Can you work these out from the model? Positions are in its coordinate system, mm. A direction names the side the tool comes from. Coordinates: 2 decimals unless noted, no trailing zeros. Order: outer loops, then holes, each group sorted by start corner. A loop starts at its lowest first (then second) coordinate and runs counter-clockwise, first axis right, second up. Notation, with made-up numbers: (-38, 41.25) -> (-16, 41.25) arc R36 cw to (-16, 75.25) -> close; hole circle Ø1 at (59, 36.5). An arc over 180 degrees is marked (long way). Return JSON: item names as keys, results as strings. Group by question number.
1) For pin 1 (8 mm diameter, centred on x = -94.5, y = 19, fed in from -Z); pin 2 (8 mm diameter, centred on y = 14.5, z = -120.5, fed in from -X); pin 3 (1.5 mm diameter, centred on x = -74.5, z = -125.5, fed in from -Y), each with a flat end and sliding along its axis, tell me the tip position at first contact or that it passes through.
2) Thinking about a two-plate mould opening in X: for faces 4 (the cylindrical face through (-73.365, 15.077, -118.443)), 5 (the flat face through (-70.9, 11, -122)), 6 (the cylindrical face through (-87.404, 15.154, -104.477)), 7 (the flat face through (-110.9, 15, -103)), which applies, +X half, -X half, draft (parallel to the pull), parting line (faces both ways), or undercut?
3) If we section it at B-B, the plane z = -124.5: Please give me the cut outline in (x, y).
4) For faces 1 (the flat face through (-75.9, 11, -125)), 2 (the flat face through (-72, 15, -141.942)), 3 (the flat face through (-73, 11.5, -127)), which set-ups out of +Z, -Z, +X, -X, +Y, -Y let a thin tool reach every point of the face, with its end or its side?
5) If we section it at A-A, the plane y = 15: Please give me the cut outline in (x, z).
6) If we section it at C-C, the plane x = -90.5: Please give me the cut outline in (y, z).
7) If we section it at D-D, the plane y = 8.5: Please give me the cut outline in (x, z), then the cut area to 3 significant figures.
8) If I drill on probe 1 along Z at (x, y) = (-73, 5.25); probe 2 along Z at (x, y) = (-88.5, 22); probe 3 along X at (y, z) = (7.75, -111.5), over which ranges is the centre line in solid material (lowest first)? Write a range as from..to.
from build123d import *

# Parameters (mm, degrees)
F1_DEPTH = 30
F3_D     = 7
F5_DEPTH = 25


with BuildPart() as f1:
    # F0 (on Front) → F1 (new body)
    with BuildSketch(Plane.XZ):
        with BuildLine():
            ThreePointArc((-80.400344, -106.942194), (-77.515036, -107.988935), (-75.972026, -110.642194))
            ThreePointArc((-75.972026, -110.642194), (-75.9183, -111.040591), (-75.900344, -111.442194))
            Line((-75.900344, -111.442194), (-75.900344, -138.942194))
            ThreePointArc((-75.900344, -138.942194), (-75.021664, -141.063514), (-72.900344, -141.942194))
            Line((-72.900344, -141.942194), (-70.900344, -141.942194))
            Line((-70.900344, -141.942194), (-70.900344, -101.942194))
            Line((-70.900344, -101.942194), (-110.900344, -101.942194))
            Line((-110.900344, -101.942194), (-110.900344, -103.942194))
            ThreePointArc((-110.900344, -103.942194), (-110.021664, -106.063514), (-107.900344, -106.942194))
            Line((-107.900344, -106.942194), (-80.400344, -106.942194))
        make_face()
    extrude(amount=-F1_DEPTH)

    # F3 (through all)
    with Locations(Plane.XY.offset(-101.942194)):
        with Locations((-90.900344, 15)):
            Hole(F3_D / 2)

    # F4 (on face) → F5 (cut)
    with BuildSketch(Plane.YZ.offset(-70.900344)):
        with BuildLine():
            ThreePointArc((11.5, -131.942194), (15, -135.442194), (18.5, -131.942194))
            Line((18.5, -131.942194), (18.5, -121.942194))
            ThreePointArc((18.5, -121.942194), (15, -118.442194), (11.5, -121.942194))
            Line((11.5, -121.942194), (11.5, -131.942194))
        make_face()
    extrude(amount=-F5_DEPTH, mode=Mode.SUBTRACT)


solid = f1.part
Result sheet:
{
 "1": {"pin 1": "stops at z = -106.94", "pin 2": "stops at x = -75.9", "pin 3": "stops at y = 0"},
 "2": {"face 4": "draft", "face 5": "+X half", "face 6": "undercut", "face 7": "-X half"},
 "3": {"outline": "(-75.9, 0) -> (-70.9, 0) -> (-70.9, 11.5) -> (-75.9, 11.5) -> close; (-75.9, 18.5) -> (-70.9, 18.5) -> (-70.9, 30) -> (-75.9, 30) -> close"},
 "4": {"face 1": "-Z, -X, +Y, -Y", "face 2": "-Z, +X, -X, +Y, -Y", "face 3": "+X, -X"},
 "5": {"outline": "(-110.9, -103.94) arc R3 ccw to (-107.9, -106.94) -> (-94.4, -106.94) -> (-94.4, -101.94) -> (-110.9, -101.94) -> close; (-87.4, -106.94) -> (-80.4, -106.94) arc R4.5 cw to (-75.97, -110.64) arc R4.5 cw to (-75.9, -111.44) -> (-75.9, -118.44) -> (-70.9, -118.44) -> (-70.9, -101.94) -> (-87.4, -101.94) -> close; (-75.9, -138.94) arc R3 ccw to (-72.9, -141.94) -> (-70.9, -141.94) -> (-70.9, -135.44) -> (-75.9, -135.44) -> close"},
 "6": {"outline": "(0, -106.94) -> (11.52, -106.94) -> (11.52, -101.94) -> (0, -101.94) -> close; (18.48, -106.94) -> (30, -106.94) -> (30, -101.94) -> (18.48, -101.94) -> close"},
 "7": {"outline": "(-110.9, -103.94) arc R3 ccw to (-107.9, -106.94) -> (-80.4, -106.94) arc R4.5 cw to (-75.97, -110.64) arc R4.5 cw to (-75.9, -111.44) -> (-75.9, -138.94) arc R3 ccw to (-72.9, -141.94) -> (-70.9, -141.94) -> (-70.9, -101.94) -> (-110.9, -101.94) -> close", "area": "375 mm2"},
 "8": {"probe 1": "z = -141.94..-101.94", "probe 2": "z = -106.94..-101.94", "probe 3": "x = -75.9..-70.9"}
}
